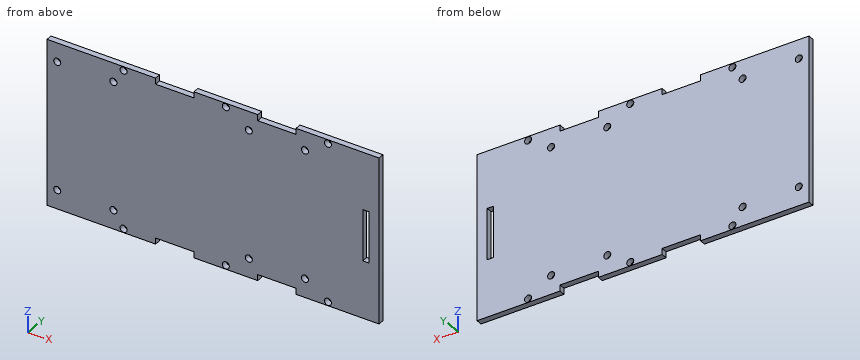
from build123d import *

# Parameters (mm, degrees)
SKETCH1_R           = 1.7526
SKETCH1_W           = 3
SKETCH1_H           = 25.4
BOSS_EXTRUDE1_DEPTH = 3
SKETCH2_R           = 1.7526
CUT_EXTRUDE1_DEPTH  = 4


with BuildPart() as part:
    # Sketch1 → Boss-Extrude1 (new body)
    with BuildSketch(Plane(origin=(0, 0, 0), x_dir=(1, 0, 0), z_dir=(0, 1, 0))):
        Polygon((-114.3, 41.1), (-77.528882775, 41.1), (-74.871117225, 41.1), (-60.325, 41.1), (-60.325, 38.1), (-41.275, 38.1), (-41.275, 41.1), (-26.728882775, 41.1), (-24.071117225, 41.1), (-9.525, 41.1), (-9.525, 38.1), (9.525, 38.1), (9.525, 41.1), (24.071117225, 41.1), (26.728882775, 41.1), (50.8, 41.1), (50.8, -41.1), (26.728882775, -41.1), (24.071117225, -41.1), (9.525, -41.1), (9.525, -38.1), (-9.525, -38.1), (-9.525, -41.1), (-24.071117225, -41.1), (-26.728882775, -41.1), (-41.275, -41.1), (-41.275, -38.1), (-60.325, -38.1), (-60.325, -41.1), (-74.871117225, -41.1), (-77.528882775, -41.1), (-114.3, -41.1), align=None)
        with Locations((-25.4, -39.195)):
            Circle(SKETCH1_R, mode=Mode.SUBTRACT)
        with Locations((25.4, -39.195)):
            Circle(SKETCH1_R, mode=Mode.SUBTRACT)
        with Locations((25.4, 39.195)):
            Circle(SKETCH1_R, mode=Mode.SUBTRACT)
        with Locations((-25.4, 39.195)):
            Circle(SKETCH1_R, mode=Mode.SUBTRACT)
        with Locations((-76.2, 39.195)):
            Circle(SKETCH1_R, mode=Mode.SUBTRACT)
        with Locations((-76.2, -39.195)):
            Circle(SKETCH1_R, mode=Mode.SUBTRACT)
        with Locations((44.22, 0)):
            Rectangle(SKETCH1_W, SKETCH1_H, mode=Mode.SUBTRACT)
    extrude(amount=BOSS_EXTRUDE1_DEPTH)

    # Sketch2 → Cut-Extrude1 (cut, through all)
    with BuildSketch(Plane(origin=(0, 3, 0), x_dir=(1, 0, 0), z_dir=(0, 1, 0))):
        with Locations((-109.22, -31.75)):
            Circle(SKETCH2_R)
        with Locations((-81.28, -31.75)):
            Circle(SKETCH2_R)
        with Locations((13.97, -31.75)):
            Circle(SKETCH2_R)
        with Locations((-13.97, -31.75)):
            Circle(SKETCH2_R)
    cut_extrude1 = extrude(amount=-CUT_EXTRUDE1_DEPTH, mode=Mode.SUBTRACT)

    # Mirror1: Cut-Extrude1 across plane
    add(cut_extrude1.mirror(Plane.XY), mode=Mode.SUBTRACT)


solid = part.part
Design review of the part built by this model. Coordinates are the model's own, in mm. Round coordinates to 2 decimals unless told otherwise and drop trailing zeros. Write each loop counter-clockwise with the first axis right and the second up, starting at its lowest first coordinate (ties: lowest second). Pieces come first, ordered by that corner, then holes. Notation, with made-up numbers: (17.25, -31.75) -> (42.25, -31.75) arc R19 ccw to (42.25, -6.75) -> close; hole circle Ø3 at (45.5, 45). An arc over 180 degrees is marked (long way). One line per item, written item: value. Start each with the question number.
Q1. Add section C-C (z = -31.75). Give the boundary of the cut face in (x, y).
Q2. Add section D-D (y = 0.65). State how many separate pieces and enclosed holes the cut face has, then the cut area to 3 significant figures.
Q3. To check wall thickness, follow probe 1 along Z at (x, y) = (-81.28, 2.15); probe 2 along X at (y, z) = (1, -31.75); probe 3 along Z at (x, y) = (-76.2, 2.35). State the ranges of each line that lie inside material, in increasing order.
Q4. Insertion check: P1, Ø4.5, axis at x = -13.97, z = 31.75, coming from the +Y side. The pin has a flat end and moves straight along its axis. Give the tip position at first contact, or say it passes through.
Q5. Add section B-B (x = -109.22). Give the boundary of the cut face in (y, z), then the cut area to 3 significant figures.
Q6. Add section A-A (z = 7). Give the boundary of the cut face in (x, y), then the cut area to 3 significant figures.
Response:
1. outline: (-114.3, 0) -> (-110.97, 0) -> (-110.97, 3) -> (-114.3, 3) -> close; (-107.47, 0) -> (-83.03, 0) -> (-83.03, 3) -> (-107.47, 3) -> close; (-79.53, 0) -> (-15.72, 0) -> (-15.72, 3) -> (-79.53, 3) -> close; (-12.22, 0) -> (12.22, 0) -> (12.22, 3) -> (-12.22, 3) -> close; (15.72, 0) -> (50.8, 0) -> (50.8, 3) -> (15.72, 3) -> close
2. separate pieces: 1
2. enclosed holes: 15
2. area: 13,100 mm^2
3. probe 1: z = -41.1 to -33.5, -30 to 30, 33.5 to 41.1
3. probe 2: x = -114.3 to -110.97, -107.47 to -83.03, -79.53 to -15.72, -12.22 to 12.22, 15.72 to 50.8
3. probe 3: z = -41.1 to -40.95, -37.44 to 37.44, 40.95 to 41.1
4. P1: stops at y = 3
5. outline: (0, -41.1) -> (3, -41.1) -> (3, -33.5) -> (0, -33.5) -> close; (0, -30) -> (3, -30) -> (3, 30) -> (0, 30) -> close; (0, 33.5) -> (3, 33.5) -> (3, 41.1) -> (0, 41.1) -> close
5. area: 226 mm^2
6. outline: (-114.3, 0) -> (42.72, 0) -> (42.72, 3) -> (-114.3, 3) -> close; (45.72, 0) -> (50.8, 0) -> (50.8, 3) -> (45.72, 3) -> close
6. area: 486 mm^2
